Input: part model. Units: mm. Frame: model coordinates. Face numbers are marked on the shaded views. A direction names the side the tool comes from. Coordinates: 2 decimals unless noted, no trailing zeros. Loops run counter-clockwise (first coordinate to the right, second up) from the corner with the lowest first, then second, coordinate; pieces in that order, holes last. Notation, with made-up numbers: (76, -7.5) - (103, -7.5) arc R32 cw to (103, 23.5) - close; hole circle Ø8 at (-22, 47.5). An arc over 180 degrees is marked (long way). Use a Markdown table: item, result. Add a question column.
1. Ray query, L1, parallel to X at y = 2, z = 20; L2, parallel to Z at x = -9.3, y = 0.6; L3, parallel to Z at x = -10, y = 67.5. Return the intervals inside material, ascending. Write a range as [from, to].
2. Section query C-C on y = 6. Return the cut outline in (x, z).
3. Section query B-B on z = 20. Return the cut outline in (x, y).
4. Contact query for flat-ended pins moving along their axis: P1, Ø1.5, axis at x = -10, y = 28, coming from the +Z side; P2, Ø1.5, axis at y = 5, z = 22, coming from the -X side; P3, Ø0.9, axis at x = 14.5, z = 19, coming from the +Y side. Output: stop coordinate, or through.
5. Section query A-A on x = 9.3. Return the cut outline in (y, z), then the cut area to 3 significant figures.
6. Section query D-D on x = -6. Return the cut outline in (y, z).
7. Access query for the marked faces 1 and 2. Directions: +Z, -Z, +X, -X, +Y, -Y. A direction counts if a zero-diameter tool reaches every point of the face in a straight line with its end or side. Return the directions, or none.
8. Draft query along X for the marked faces 3, 4, 5 and 6. Return one class per face: released by +X, released by -X, zero draft, split by the parting line, or undercut.
Autodesk Inventor part; units mm, degrees
ref_plane "YZ Plane" through (0, 0, 0) normal (1, 0, 0) x (0, 1, 0)
ref_plane "XZ Plane" through (0, 0, 0) normal (0, 1, 0) x (-1, 0, 0)
ref_plane "XY Plane" through (0, 0, 0) normal (0, 0, 1) x (1, 0, 0)
sketch "スケッチ1" plane through (0, 0, 0) normal (0, 1, 0) x (-1, 0, 0)
  line L0 (30, 15) -> (-30, 15)
  line L1 (-30, 15) -> (-30, -15)
  line L2 (-30, -15) -> (30, -15)
  line L3 (30, -15) -> (30, 15)
  line L4 (30, 15) -> (-30, -15) construction
  line L5 (-30, 15) -> (30, -15) construction
  point P0 (0, 0)
  dimension "d0" = 60
  dimension "d1" = 30
extrude "押し出し1" add sketch "スケッチ1" along normal blind 85
sketch "スケッチ2" plane through (0, 0, 0) normal (0, -1, 0) x (1, 0, 0)
  line L0 (16, 5) -> (-16, 5)
  line L1 (-16, 5) -> (-16, 25)
  line L2 (-16, 25) -> (16, 25)
  line L3 (16, 25) -> (16, 5)
  line L4 (-30, 15) -> (30, 15)
  line L5 (16, 5) -> (-16, 25) construction
  line L6 (-16, 5) -> (16, 25) construction
  point P0 (0, 0)
  point P1 (0, 15)
  point P2 (-16, 15)
  point P3 (16, 15)
  dimension "d4" = 32
  dimension "d5" = 20
extrude "押し出し2" add sketch "スケッチ2" against normal blind 3 contours L4 L1 L2 L3
sketch "スケッチ3" plane through (0, 3, 0) normal (0, 1, 0) x (1, 0, 0)
  line L0 (-16, -25) -> (16, -25)
  line L1 (-30, -15) -> (30, -15)
  line L2 (16, -25) -> (13, -25)
  line L3 (13, -25) -> (13, -15)
  line L4 (13, -15) -> (16, -15)
  line L5 (16, -15) -> (16, -25)
  line L6 (-16, -15) -> (-16, -25)
  line L7 (-16, -25) -> (-13, -25)
  line L8 (-13, -25) -> (-13, -15)
  line L9 (-13, -15) -> (-16, -15)
  line L10 (-16, -15) -> (-16, -25)
  point P0 (0, 0)
  point P1 (-13, -25)
  point P2 (-13, -15)
  point P3 (16, -15)
  dimension "d8" = 3
  dimension "d9" = 3
extrude "押し出し3" add sketch "スケッチ3" along normal blind 5 contours L6 L1 L8 L0 | L3 L1 L5 L0
sketch "スケッチ4" plane through (0, 3, 0) normal (0, 1, 0) x (1, 0, 0)
  line L0 (13, -25) -> (16, -25)
  line L1 (-13, -15) -> (-13, -25)
  line L2 (13, -25) -> (-13, -25)
  line L3 (-13, -25) -> (-13, -20)
  line L4 (-13, -20) -> (13, -20)
  line L5 (13, -20) -> (13, -25)
  line L6 (-13, -15) -> (13, -15)
  line L7 (9.3, -25) -> (-9.3, -25)
  line L8 (-9.3, -25) -> (-9.3, -15)
  line L9 (-9.3, -15) -> (9.3, -15)
  line L10 (9.3, -15) -> (9.3, -25)
  line L11 (9.3, -25) -> (-9.3, -15) construction
  line L12 (-9.3, -25) -> (9.3, -15) construction
  point P0 (0, 0)
  point P1 (0, -20)
  point P2 (9.3, -20)
  point P3 (-9.3, -20)
  dimension "d12" = 5
  dimension "d13" = 18.6
hole "穴1" at (9.3, 3, 20) at (-9.3, 3, 20) direction (0, -1, 0) diameter 4 end through all
properties part number "_3D プリント"
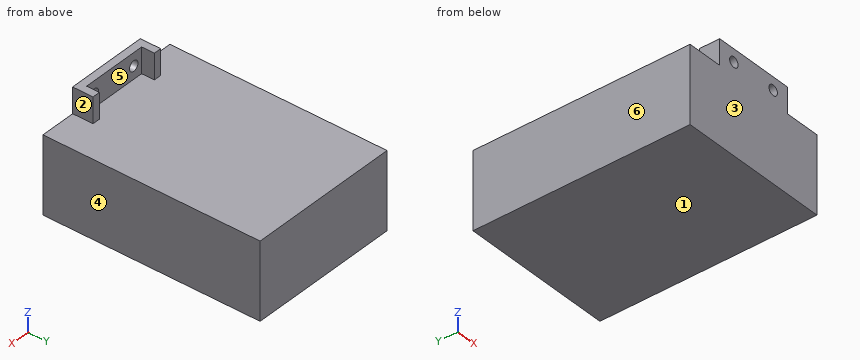
Resolved:
| question | item | result |
|---|---|---|
| 1 | L1 | [-16, -11.3], [-7.3, 7.3], [11.3, 16] |
| 1 | L2 | [-15, 18], [22, 25] |
| 1 | L3 | [-15, 15] |
| 2 | outline | (-30, -15) - (30, -15) - (30, 15) - (16, 15) - (16, 25) - (13, 25) - (13, 15) - (-13, 15) - (-13, 25) - (-16, 25) - (-16, 15) - (-30, 15) - close |
| 3 | outline | (-16, 0) - (-11.3, 0) - (-11.3, 3) - (-13, 3) - (-13, 8) - (-16, 8) - close; (-7.3, 0) - (7.3, 0) - (7.3, 3) - (-7.3, 3) - close; (11.3, 0) - (16, 0) - (16, 8) - (13, 8) - (13, 3) - (11.3, 3) - close |
| 4 | P1 | z = 15 |
| 4 | P2 | x = -16 |
| 4 | P3 | y = 8 |
| 5 | outline | (0, -15) - (85, -15) - (85, 15) - (3, 15) - (3, 18) - (0, 18) - close; (0, 22) - (3, 22) - (3, 25) - (0, 25) - close |
| 5 | area | 2,570 mm² |
| 6 | outline | (0, -15) - (85, -15) - (85, 15) - (3, 15) - (3, 25) - (0, 25) - close |
| 7 | face 1 | -Z, +X, -X, +Y, -Y |
| 7 | face 2 | +Z, +X, +Y, -Y |
| 8 | face 3 | zero draft |
| 8 | face 4 | released by +X |
| 8 | face 5 | undercut |
| 8 | face 6 | released by -X |
